The figure shows three views and two pictorial views of one solid part (mm, origin at its lowest corner). Answer the questions. A direction names the side the tool comes from. Give positions to 0.01 mm unless a question says otherwise; leave off trailing zeros. Order: outer loops, then holes, each group sorted by start corner. A loop starts at its lowest first (then second) coordinate and runs counter-clockwise, first axis right, second up. Notation, with made-up numbers: M 64,79 L 106,79 A26 cw 106,115 Z; hole C -15,22.5 d11. An arc over 180 degrees is marked long. One line per item, written item: value.
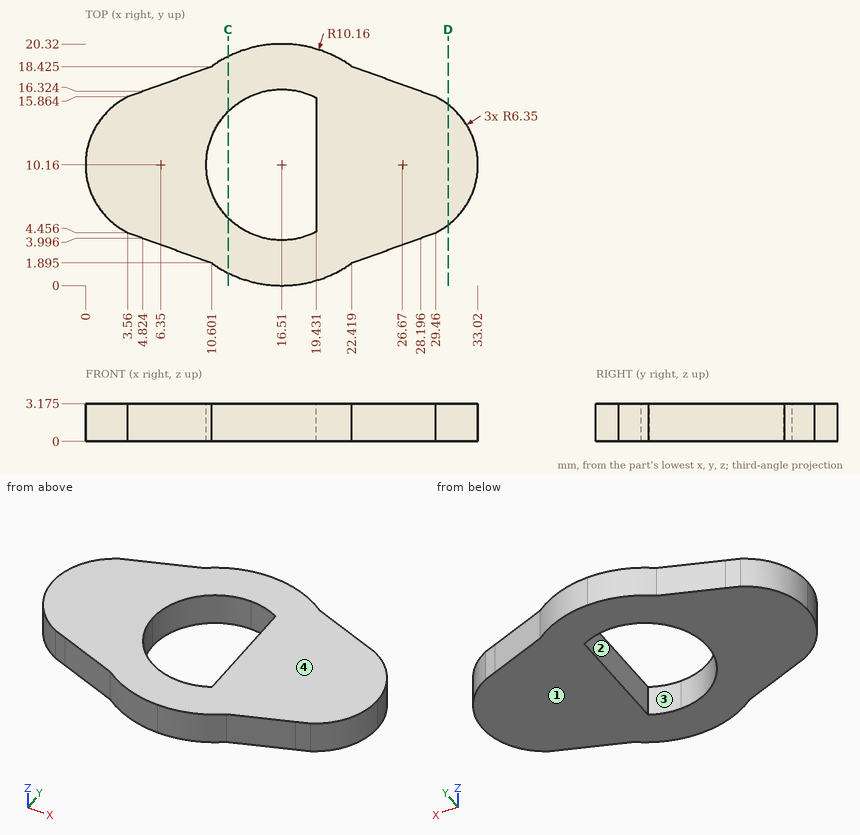
1) Find section D-D, the plane x = 30.5. Write down the section's boundary in (y, z) (1 decimal).
Reported:
outline: M 5.1,0 L 15.2,0 L 15.2,3.2 L 5.1,3.2 Z
2) Each of these flat-tipped pins is pushed along its axis until it touches: pin 1 Ø1.5 at (y, z) = (4.5, 0.5) entering from -X (1 decimal); pin 2 Ø1.6 at (y, z) = (10.5, 2) entering from -X; pin 3 Ø1.5 at (y, z) = (9, 1.5) entering from +X. Where does it stop, or does it pass through?
Reported:
pin 1: stops at x = 2.3
pin 2: stops at x = 0
pin 3: stops at x = 33.01
3) Which of the six approach directions +Z, -Z, +X, -X, +Y, -Y give full straight-line access (tool end or side, diameter ignored) to the marked faces 1 and 2?
Reported:
face 1: -Z, +X, -X, +Y, -Y
face 2: +Z, -Z
4) Consider probe 1 along X at (y, z) = (11.75, 1.35); probe 2 along X at (y, z) = (14, 0.55) (1 decimal); probe 3 along Y at (x, z) = (30, 1.15) (1 decimal). Determine where each line is inside the solid, lowest interval first.
Reported:
probe 1: x = 0.2 to 10.36, 19.43 to 32.82
probe 2: x = 1.3 to 11.5, 19.4 to 31.7
probe 3: y = 4.8 to 15.6
5) Determine the mould class of the marked faces 3 and 4 for opening direction Y: +Y half, -Y half, draft (parallel to the pull), parting line (faces both ways), or undercut.
Reported:
face 3: undercut
face 4: draft
6) Find section C-C, the plane x = 12. Write down the section's boundary in (y, z) (1 decimal).
Reported:
outline: M 1.1,0 L 5.7,0 L 5.7,3.2 L 1.1,3.2 Z; M 14.6,0 L 19.3,0 L 19.3,3.2 L 14.6,3.2 Z
